from build123d import *

# Parameters (mm, degrees)
SKETCH_1_W          = 1
SKETCH_1_H          = 120
EXTRUDE_1_DEPTH     = 20
SKETCH_2_R          = 1.8
CUT_EXTRUDE_1_DEPTH = 122.659360511
SKETCH_3_R          = 1.8
CUT_EXTRUDE_3_DEPTH = 10
SKETCH_4_R          = 1.8
CUT_EXTRUDE_4_DEPTH = 122.659360511


with BuildPart() as part:
    # 草图1 → 凸台-拉伸1 (new body)
    with BuildSketch(Plane(origin=(0, 0, 0), x_dir=(1, 0, 0), z_dir=(0, 1, 0))):
        with Locations((0.5, 60)):
            Rectangle(SKETCH_1_W, SKETCH_1_H)
    extrude(amount=EXTRUDE_1_DEPTH)

    # 草图2 → 切除-拉伸1 (cut, through all)
    with BuildSketch(Plane.ZY):
        with Locations((-10, 17)):
            Circle(SKETCH_2_R)
        with Locations((-17, 10)):
            Circle(SKETCH_2_R)
        with Locations((-3, 10)):
            Circle(SKETCH_2_R)
        with Locations((-10, 3)):
            Circle(SKETCH_2_R)
    extrude(amount=-CUT_EXTRUDE_1_DEPTH, mode=Mode.SUBTRACT)

    # 草图3 → 切除-拉伸3 (cut)
    with BuildSketch(Plane.ZY):
        with Locations((-110, 10)):
            Circle(SKETCH_3_R)
        with Locations((-95, 10)):
            Circle(SKETCH_3_R)
        with Locations((-80, 10)):
            Circle(SKETCH_3_R)
        with Locations((-65, 10)):
            Circle(SKETCH_3_R)
    extrude(amount=-CUT_EXTRUDE_3_DEPTH, mode=Mode.SUBTRACT)

    # 草图4 → 切除-拉伸4 (cut, through all)
    with BuildSketch(Plane.ZY):
        with Locations((-28, 16)):
            Circle(SKETCH_4_R)
        with Locations((-28, 4)):
            Circle(SKETCH_4_R)
    extrude(amount=-CUT_EXTRUDE_4_DEPTH, mode=Mode.SUBTRACT)


solid = part.part
Can you work these out from the model? Positions are in its coordinate system, mm. Coordinates: 2 decimals unless noted, no trailing zeros. Write each loop counter-clockwise with the first axis right and the second up, starting at its lowest first coordinate (ties: lowest second). Pieces come first, ordered by that corner, then holes. Notation, with made-up numbers: (-5, 84.25) -> (26, 84.25) arc R14 ccw to (26, 100.25) -> close; hole circle Ø6 at (38, -4). An arc over 180 degrees is marked (long way). Write each question's results on one line, items separated by ' | '. Start each with the question number.
Q1. I'm going to push a flat-ended pin straight in: pin 1 (4 mm diameter, centred on y = 4, z = -28, fed in from +X). Where does the tip first touch, or does it pass through?
Q2. Imagine slicing it at C-C (x = 0.45). State how many separate pieces and enclosed holes the cut face has, then the cut area to 3 significant figures.
Q3. Imagine slicing it at B-B (y = 10). Write out the boundary of the cut face in (x, z).
Q4. If I drill on probe 1 along Y at (x, z) = (0.6, -3); probe 2 along Z at (x, y) = (0.1, 2.75); probe 3 along Z at (x, y) = (0.5, 17.5), over which ranges is the centre line in solid material (lowest first)?
Q5. Imagine slicing it at A-A (z = -80). Write out the boundary of the cut face in (x, y), then the cut area to 3 significant figures.
Q6. We'd pull the mould along Y, two halves only. Please class faces 1 (the face through (0.493, 8.243, -17.39)), 2 (the face through (0, 10, -59)): +Y half, -Y half, draft (parallel to the pull), parting line (faces both ways), or undercut.
Taken from the geometry:
1) pin 1: stops at x = 1
2) separate pieces: 1 | enclosed holes: 10 | area: 2,300 mm^2
3) outline: (0, -120) -> (1, -120) -> (1, -111.8) -> (0, -111.8) -> close; (0, -108.2) -> (1, -108.2) -> (1, -96.8) -> (0, -96.8) -> close; (0, -93.2) -> (1, -93.2) -> (1, -81.8) -> (0, -81.8) -> close; (0, -78.2) -> (1, -78.2) -> (1, -66.8) -> (0, -66.8) -> close; (0, -63.2) -> (1, -63.2) -> (1, -18.8) -> (0, -18.8) -> close; (0, -15.2) -> (1, -15.2) -> (1, -4.8) -> (0, -4.8) -> close; (0, -1.2) -> (1, -1.2) -> (1, 0) -> (0, 0) -> close
4) probe 1: y = 0 to 8.2, 11.8 to 20 | probe 2: z = -120 to -29.3, -26.7 to -11.78, -8.22 to 0 | probe 3: z = -120 to -28.99, -27.01 to -11.73, -8.27 to 0
5) outline: (0, 0) -> (1, 0) -> (1, 8.2) -> (0, 8.2) -> close; (0, 11.8) -> (1, 11.8) -> (1, 20) -> (0, 20) -> close | area: 16.4 mm^2
6) face 1: undercut | face 2: draft
